Read the model definition and answer for the solid it produces. Units are mm, in the model's axes. Give positions to 0.01 mm unless a question says otherwise; leave off trailing zeros. Order: outer loops, then holes, each group sorted by start corner. A loop starts at its lowest first (then second) coordinate and runs counter-clockwise, first axis right, second up. Notation, with made-up numbers: M -4,20.5 L 11,20.5 A13 cw 11,32.5 Z; hole C 22,20.5 d5. An arc over 180 degrees is marked long. One line per item, written item: value.
from build123d import *

# Parameters (mm, degrees)
F1_DEPTH = 6.35
F3_D     = 28.575


# Not quite as in the source:
# - a feature names something its author has since deleted; it is built from what else it names


with BuildPart() as f1:
    # F0 (on Top) → F1 (new body)
    with BuildSketch(Plane.XY):
        with BuildLine():
            Line((-914.4, 0), (0, 0))
            Line((0, 0), (0, 304.8))
            ThreePointArc((0, 304.8), (-7.2393593738, 330.9363843757), (-26.8941176471, 349.6235294118))
            ThreePointArc((-26.8941176471, 349.6235294118), (-457.2, 457.2), (-887.5058823529, 349.6235294118))
            ThreePointArc((-887.5058823529, 349.6235294118), (-907.1606406262, 330.9363843757), (-914.4, 304.8))
            Line((-914.4, 304.8), (-914.4, 0))
        make_face()
    extrude(amount=F1_DEPTH)

    # F3 (through all)
    with Locations(Plane(origin=(0, 0, 0), x_dir=(1, 0, 0), z_dir=(0, 0, -1))):
        with Locations((-415.925, -50.8), (-374.65, -50.8), (-457.2, -50.8), (-498.475, -50.8), (-539.75, -50.8)):
            Hole(F3_D / 2)


solid = f1.part
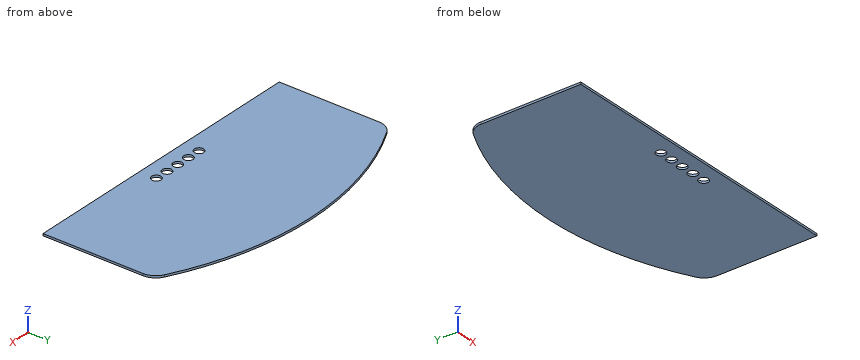
1) Find section A-A, the plane y = 50.8. Write down the section's boundary in (x, z).
Reported:
outline: M -914.4,0 L -554.04,0 L -554.04,6.35 L -914.4,6.35 Z; M -525.46,0 L -512.76,0 L -512.76,6.35 L -525.46,6.35 Z; M -484.19,0 L -471.49,0 L -471.49,6.35 L -484.19,6.35 Z; M -442.91,0 L -430.21,0 L -430.21,6.35 L -442.91,6.35 Z; M -401.64,0 L -388.94,0 L -388.94,6.35 L -401.64,6.35 Z; M -360.36,0 L 0,0 L 0,6.35 L -360.36,6.35 Z
2) Consider probe 1 along X at (y, z) = (50.8, 4); probe 2 along X at (y, z) = (45, 4.25); probe 3 along Y at (x, z) = (-374.65, 2.5). Determine where each line is inside the solid, lowest interval first.
Reported:
probe 1: x = -914.4 to -554.04, -525.46 to -512.76, -484.19 to -471.49, -442.91 to -430.21, -401.64 to -388.94, -360.36 to 0
probe 2: x = -914.4 to -552.81, -526.69 to -511.53, -485.42 to -470.26, -444.14 to -428.98, -402.87 to -387.71, -361.59 to 0
probe 3: y = 0 to 36.51, 65.09 to 453.47
3) Find section D-D, the plane x = -129. Write down the section's boundary in (y, z).
Reported:
outline: M 0,0 L 396.27,0 L 396.27,6.35 L 0,6.35 Z
4) Find section C-C, the plane z = 4.25. Count the separate pieces of the cut face and the enclosed holes in it, plus the area to 3 significant figures.
Reported:
separate pieces: 1
enclosed holes: 5
area: 378,000 mm^2
5) Find section B-B, the plane x = -457.2. Write down the section's boundary in (y, z), plus the area to 3 significant figures.
Reported:
outline: M 0,0 L 36.51,0 L 36.51,6.35 L 0,6.35 Z; M 65.09,0 L 457.2,0 L 457.2,6.35 L 65.09,6.35 Z
area: 2,720 mm^2
